Autodesk Inventor part; units mm, degrees
ref_plane "YZ Plane" through (0, 0, 0) normal (1, 0, 0) x (0, 1, 0)
ref_plane "XZ Plane" through (0, 0, 0) normal (0, 1, 0) x (-1, 0, 0)
ref_plane "XY Plane" through (0, 0, 0) normal (0, 0, 1) x (1, 0, 0)
sketch "Sketch1" plane through (0, 0, 0) normal (0, 0, 1) x (1, 0, 0)
  line L0 (-34.86, 0) -> (34.86, 0) construction
  line L1 (0, -34.86) -> (0, 34.86) construction
  line L2 (0, 0) -> (11.1575, 11.1575) construction
  line L3 (0, 0) -> (15.7791, 0) construction
  line L4 (0, 24.9) -> (16.8009, 24.9)
  line L5 (16.8009, 24.9) -> (16.8009, 21.2415)
  line L6 (16.8009, 21.2415) -> (19.0212, 19.0212)
  line L7 (24.9, 0) -> (24.9, 16.8009)
  line L8 (24.9, 16.8009) -> (21.2415, 16.8009)
  line L9 (21.2415, 16.8009) -> (19.0212, 19.0212)
  line L10 (0, -24.9) -> (16.8009, -24.9)
  line L11 (16.8009, -24.9) -> (16.8009, -21.2415)
  line L12 (16.8009, -21.2415) -> (19.0212, -19.0212)
  line L13 (24.9, 0) -> (24.9, -16.8009)
  line L14 (24.9, -16.8009) -> (21.2415, -16.8009)
  line L15 (21.2415, -16.8009) -> (19.0212, -19.0212)
  line L16 (0, 24.9) -> (-16.8009, 24.9)
  line L17 (-16.8009, 24.9) -> (-16.8009, 21.2415)
  line L18 (-16.8009, 21.2415) -> (-19.0212, 19.0212)
  line L19 (-24.9, 16.8009) -> (-21.2415, 16.8009)
  line L20 (-21.2415, 16.8009) -> (-19.0212, 19.0212)
  line L21 (0, -24.9) -> (-16.8009, -24.9)
  line L22 (-16.8009, -24.9) -> (-16.8009, -21.2415)
  line L23 (-16.8009, -21.2415) -> (-19.0212, -19.0212)
  line L24 (-21.2415, -16.8009) -> (-19.0212, -19.0212)
  line L25 (-24.9, -16.8009) -> (-21.2415, -16.8009)
  line L26 (-24.9, 0) -> (-24.9, -16.8009)
  line L27 (-24.9, 0) -> (-24.9, 16.8009)
  circle A0 centre (0, 0) radius 12.5
  dimension "d0" = 45
  dimension "d2" = 24.9
  dimension "d3" = 3.14
  dimension "d4" = 26.9
  dimension "d5" = 25
extrude "Extrusion1" add sketch "Sketch1" along normal blind 5
sketch "Sketch2" plane through (0, 0, 5) normal (0, 0, 1) x (1, 0, 0)
  circle A0 centre (0, 0) radius 12.5
  line L0 (16.8009, 24.9) -> (-16.8009, 24.9)
  line L1 (-16.8009, 24.9) -> (-16.8009, 21.2415)
  line L2 (-16.8009, 21.2415) -> (-21.2415, 16.8009)
  line L3 (-21.2415, 16.8009) -> (-24.9, 16.8009)
  line L4 (-24.9, 16.8009) -> (-24.9, -16.8009)
  line L5 (-24.9, -16.8009) -> (-21.2415, -16.8009)
  line L6 (-21.2415, -16.8009) -> (-16.8009, -21.2415)
  line L7 (-16.8009, -21.2415) -> (-16.8009, -24.9)
  line L8 (-16.8009, -24.9) -> (16.8009, -24.9)
  line L9 (16.8009, -24.9) -> (16.8009, -21.2415)
  line L10 (16.8009, -21.2415) -> (21.2415, -16.8009)
  line L11 (21.2415, -16.8009) -> (24.9, -16.8009)
  line L12 (24.9, -16.8009) -> (24.9, 16.8009)
  line L13 (24.9, 16.8009) -> (21.2415, 16.8009)
  line L14 (21.2415, 16.8009) -> (16.8009, 21.2415)
  line L15 (16.8009, 21.2415) -> (16.8009, 24.9)
  line L16 (-34.86, 0) -> (34.86, 0) construction
  line L17 (0, -34.86) -> (0, 34.86) construction
  line L18 (-10, 21.9) -> (10, 21.9)
  line L19 (10, 21.9) -> (10, 18.9)
  line L20 (10, 18.9) -> (-10, 18.9)
  line L21 (-10, 18.9) -> (-10, 21.9)
  line L22 (-10, -21.9) -> (10, -21.9)
  line L23 (10, -21.9) -> (10, -18.9)
  line L24 (10, -18.9) -> (-10, -18.9)
  line L25 (-10, -18.9) -> (-10, -21.9)
  dimension "d8" = 20
  dimension "d9" = 3
  dimension "d10" = 3
extrude "Extrusion2" add sketch "Sketch2" along normal blind 7 contours L18 L19 L20 L21 | L25 L24 L23 L22
chamfer "Fase1" [suppressed]
chamfer "Fase2" [suppressed]
sketch "Sketch4" plane through (0, 0, 0) normal (0, 0, -1) x (-1, 0, 0)
  circle A0 centre (0, 0) radius 12.5 construction
  line L0 (16.8009, 24.9) -> (-16.8009, 24.9) construction
  line L1 (-16.8009, 24.9) -> (-16.8009, 21.2415)
  line L2 (-16.8009, 21.2415) -> (-21.2415, 16.8009)
  line L3 (-21.2415, 16.8009) -> (-24.9, 16.8009)
  line L4 (-24.9, 16.8009) -> (-24.9, -16.8009) construction
  line L5 (-24.9, -16.8009) -> (-21.2415, -16.8009)
  line L6 (-21.2415, -16.8009) -> (-16.8009, -21.2415)
  line L7 (-16.8009, -21.2415) -> (-16.8009, -24.9)
  line L8 (-16.8009, -24.9) -> (16.8009, -24.9) construction
  line L9 (16.8009, -24.9) -> (16.8009, -21.2415)
  line L10 (16.8009, -21.2415) -> (21.2415, -16.8009)
  line L11 (21.2415, -16.8009) -> (24.9, -16.8009)
  line L12 (24.9, -16.8009) -> (24.9, 16.8009) construction
  line L13 (24.9, 16.8009) -> (21.2415, 16.8009)
  line L14 (21.2415, 16.8009) -> (16.8009, 21.2415)
  line L15 (16.8009, 21.2415) -> (16.8009, 24.9)
  line L16 (-16.9009, 25) -> (16.9009, 25) construction
  line L17 (16.9009, 25) -> (16.9009, 21.2829)
  line L18 (16.9009, 21.2829) -> (21.2829, 16.9009)
  line L19 (21.2829, 16.9009) -> (25, 16.9009)
  line L20 (25, 16.9009) -> (25, -16.9009) construction
  line L21 (25, -16.9009) -> (21.2829, -16.9009)
  line L22 (21.2829, -16.9009) -> (16.9009, -21.2829)
  line L23 (16.9009, -21.2829) -> (16.9009, -25)
  line L24 (16.9009, -25) -> (-16.9009, -25) construction
  line L25 (-16.9009, -25) -> (-16.9009, -21.2829)
  line L26 (-16.9009, -21.2829) -> (-21.2829, -16.9009)
  line L27 (-21.2829, -16.9009) -> (-25, -16.9009)
  line L28 (-25, -16.9009) -> (-25, 16.9009) construction
  line L29 (-25, 16.9009) -> (-21.2829, 16.9009)
  line L30 (-21.2829, 16.9009) -> (-16.9009, 21.2829)
  line L31 (-16.9009, 21.2829) -> (-16.9009, 25)
  line L32 (-24.9, -16.8009) -> (-24.9, 16.8009)
  line L33 (-24.9, 16.8009) -> (-24.9, 16.9009)
  line L34 (-16.8009, 24.9) -> (-16.9009, 24.9)
  line L35 (-16.8009, 24.9) -> (16.8009, 24.9)
  line L36 (16.8009, 24.9) -> (16.9009, 24.9)
  line L37 (24.9, 16.8009) -> (24.9, 16.9009)
  line L38 (24.9, 16.8009) -> (24.9, -16.8009)
  line L39 (24.9, -16.8009) -> (24.9, -16.9009)
  line L40 (16.8009, -24.9) -> (-16.8009, -24.9)
  line L41 (16.8009, -24.9) -> (16.9009, -24.9)
  line L42 (-16.8009, -24.9) -> (-16.9009, -24.9)
  line L43 (-24.9, -16.8009) -> (-24.9, -16.9009)
  dimension "d19" = 0.1
extrude "IM_offset" add sketch "Sketch4" against normal up to surface (5 mm away) contours L1 L2 L3 L33 L29 L30 L31 L34 | L36 L17 L18 L19 L37 L13 L14 L15 | L5 L6 L7 L42 L25 L26 L27 L43 | L39 L21 L22 L23 L41 L9 L10 L11
properties part number "20_Cube_insert_Sample_holder_v3"
Source: CAD feature listing. Evaluate the final solid. Frame: model axes, mm. A direction names the side the tool comes from. Coordinates: 2 decimals unless noted, no trailing zeros. Loops run counter-clockwise (first coordinate to the right, second up) from the corner with the lowest first, then second, coordinate; pieces in that order, holes last. Notation, with made-up numbers: (20, -40) - (35, -40) arc R9 ccw to (35, -33) - close; hole circle Ø3 at (16, -17.75). An arc over 180 degrees is marked (long way). One line per item, written item: value. Start each with the question number.
1. Contact query for flat-ended pins moving along their axis: P1, Ø5.5, axis at x = 2.5, z = 10, coming from the +Y side; P2, Ø3, axis at y = -23, z = 3, coming from the +X side; P3, Ø3.5, axis at y = 20.5, z = 7.5, coming from the -X side. Output: stop coordinate, or through.
2. Section B-B (y = 0). Return the cut outline in (x, z).
3. Set-up query: faces 1 (the flat face through (0, 21.9, 8)), 2 (the flat face through (-23, 16.901, 2)), 3 (the flat face through (-16.901, -23, 2)). Return all of +Z, -Z, +X, -X, +Y, -Y with unobstructed straight access to the full face (end or side cutting, diameter ignored); none if empty.
4. Mould query, pull axis Y, two halves, no side actions, for faces 4 (the flat face through (0, -21.9, 8)), 5 (the flat face through (-10, -20, 8)), 6 (the flat face through (0, -18.9, 8)), 7 (the flat face through (0, 18.9, 8)). Classes: pulls with the +Y half, pulls with the -Y half, needs draft (parallel to the pull), parting line crosses it, or undercut.
5. Section D-D (y = 15.5). Return the cut outline in (x, z), and give its area (3 significant figures).
6. Ray query, L1, parallel to Y at x = 0, z = 2.3; L2, parallel to Y at x = 9, z = 10; L3, parallel to Z at x = 19.5, y = -15. Return the intervals inside material, ascending.
7. Section A-A (x = 0). Return the cut outline in (y, z).
8. Section C-C (z = 4.25). Return the cut outline in (x, y).
Verdict:
1. P1: stops at y = 21.9
1. P2: stops at x = 16.9
1. P3: stops at x = -10
2. outline: (-24.9, 0) - (-12.5, 0) - (-12.5, 5) - (-24.9, 5) - close; (12.5, 0) - (24.9, 0) - (24.9, 5) - (12.5, 5) - close
3. face 1: +Z, +X, -X, +Y
3. face 2: +Z, -Z, -X, +Y
3. face 3: +Z, -Z, -X, -Y
4. face 4: pulls with the -Y half
4. face 5: needs draft
4. face 6: undercut
4. face 7: undercut
5. outline: (-24.9, 0) - (24.9, 0) - (24.9, 5) - (-24.9, 5) - close
5. area: 249 mm2
6. L1: y = -24.9 to -12.5, 12.5 to 24.9
6. L2: y = -21.9 to -18.9, 18.9 to 21.9
6. L3: z = 0 to 5
7. outline: (-24.9, 0) - (-12.5, 0) - (-12.5, 5) - (-18.9, 5) - (-18.9, 12) - (-21.9, 12) - (-21.9, 5) - (-24.9, 5) - close; (12.5, 0) - (24.9, 0) - (24.9, 5) - (21.9, 5) - (21.9, 12) - (18.9, 12) - (18.9, 5) - (12.5, 5) - close
8. outline: (-24.9, -16.9) - (-21.28, -16.9) - (-16.9, -21.28) - (-16.9, -24.9) - (16.9, -24.9) - (16.9, -21.28) - (21.28, -16.9) - (24.9, -16.9) - (24.9, 16.9) - (21.28, 16.9) - (16.9, 21.28) - (16.9, 24.9) - (-16.9, 24.9) - (-16.9, 21.28) - (-21.28, 16.9) - (-24.9, 16.9) - close; hole circle Ø25 at (0, 0)
